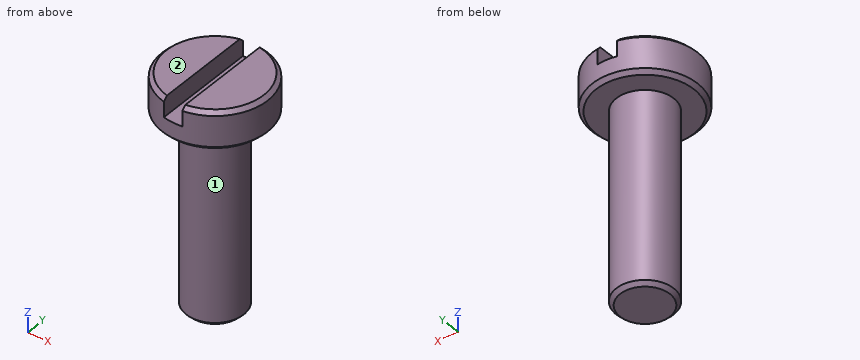
Autodesk Inventor part; units mm, degrees
ref_plane "YZ Plane" through (0, 0, 0) normal (1, 0, 0) x (0, 1, 0)
ref_plane "XZ Plane" through (0, 0, 0) normal (0, 1, 0) x (-1, 0, 0)
ref_plane "XY Plane" through (0, 0, 0) normal (0, 0, 1) x (1, 0, 0)
sketch "Náčrt1" plane through (0, 0, 0) normal (0, 0, 1) x (1, 0, 0)
  circle A0 centre (0, 0) radius 2.75
  dimension "d0" = 5.5
extrude "Vysunutí1" add sketch "Náčrt1" along normal blind 2
chamfer "Zkosení1" distance 0.2 angle 45 1 edges at (-2.75, 0, 2)
chamfer "Zkosení2" distance 0.2 angle 45 1 edges at (-2.75, 0, 0)
sketch "Náčrt2" plane through (0, 0, 2) normal (0, 0, 1) x (1, 0, 0)
  line L0 (-0.6097, -6) -> (0.3903, -6)
  line L1 (0.3903, -6) -> (0.3903, 6)
  line L2 (0.3903, 6) -> (-0.6097, 6)
  line L3 (-0.6097, 6) -> (-0.6097, -6)
  line L4 (-0.6097, -6) -> (0.3903, 6) construction
  line L5 (0.3903, -6) -> (-0.6097, 6) construction
  point P0 (0, 0)
  point P1 (-0.1097, 0)
  dimension "d9" = 1
extrude "Vysunutí2" cut sketch "Náčrt2" against normal blind 1
sketch "Náčrt3" plane through (0, 0, 0) normal (0, 0, -1) x (-1, 0, 0)
  circle A0 centre (0, 0) radius 1.5
  dimension "d12" = 3
extrude "Vysunutí3" add sketch "Náčrt3" along normal blind 10
chamfer "Zkosení3" distance 0.2 angle 45 1 edges at (1.5, 0, -10)
thread "Závit1"
properties part number "Bolt-M3x10" material "Ocel, vysokopevnostní, nízkolegovaná"
Can you work these out from the model? Positions are in its coordinate system, mm. Face numbers are marked on the shaded views. A direction names the side the tool comes from. Round coordinates to 2 decimals unless told otherwise and drop trailing zeros. Order: outer loops, then holes, each group sorted by start corner. A loop starts at its lowest first (then second) coordinate and runs counter-clockwise, first axis right, second up. Notation, with made-up numbers: (79, -9) - (108, -9) arc R19 cw to (108, 13) - close; hole circle Ø1 at (40.5, -14.75). An arc over 180 degrees is marked (long way). Answer in a Markdown table with one row per item.
(1) Suppose I cut it at B-B, the plane x = 0. Please give me the cut outline in (y, z), plus the area to 3 significant figures.
From the geometry:
| item | result |
|---|---|
| outline | (-2.75, 0.2) - (-2.55, 0) - (-1.5, 0) - (-1.5, -9.8) - (-1.3, -10) - (1.3, -10) - (1.5, -9.8) - (1.5, 0) - (2.55, 0) - (2.75, 0.2) - (2.75, 1) - (-2.75, 1) - close |
| area | 35.4 mm2 |
(2) Suppose I cut it at A-A, the plane y = 0. Please give me the cut outline in (x, z).
From the geometry:
| item | result |
|---|---|
| outline | (-2.75, 0.2) - (-2.55, 0) - (-1.5, 0) - (-1.5, -9.8) - (-1.3, -10) - (1.3, -10) - (1.5, -9.8) - (1.5, 0) - (2.55, 0) - (2.75, 0.2) - (2.75, 1.8) - (2.55, 2) - (0.39, 2) - (0.39, 1) - (-0.61, 1) - (-0.61, 2) - (-2.55, 2) - (-2.75, 1.8) - close |
(3) Suppose I cut it at C-C, the plane z = -5. Please give me the cut outline in (x, y).
From the geometry:
| item | result |
|---|---|
| outline | circle Ø3 at (0, 0) |
(4) Please list where these lines run through material, in increasing order: L1, parallel to Y at x = 0, z = -6.25; L2, parallel to Z at x = 0.35, y = -0.65; L3, parallel to Z at x = -1.6, y = 1.15. Write a range as from..to.
From the geometry:
| item | result |
|---|---|
| L1 | y = -1.5..1.5 |
| L2 | z = -10..1 |
| L3 | z = 0..2 |
(5) For P1, Ø1.5, axis at x = -0.5, z = -1.5, coming from the +Y side; P2, Ø2, axis at x = -2, z = -1.5, coming from the -Y side, each with a flat end and sliding along its axis, tell me the tip position at first contact or that it passes through.
From the geometry:
| item | result |
|---|---|
| P1 | stops at y = 1.5 |
| P2 | stops at y = -1.12 |
(6) Which directions (+Z, -Z, +X, -X, +Y, -Y) give clear straight access to the entire face, cutting with the end or side of a thin tool? Please do the marked faces 1 and 2.
From the geometry:
| item | result |
|---|---|
| face 1 | -Z |
| face 2 | +Z, +X, -X, +Y, -Y |
